Autodesk Fusion 360 part; units mm, degrees
sketch "Sketch1" plane through (0, 0, 0) normal (0, 0, 1) x (1, 0, 0)
  circle A0 centre (0, 0) radius 16.5
  circle A1 centre (0, 0) radius 15.5
  line L0 (-25, -5) -> (25, -5)
  line L1 (25, -5) -> (25, 5)
  line L2 (25, 5) -> (-25, 5)
  line L3 (-25, 5) -> (-25, -5)
  line L4 (-25, -5) -> (25, 5) construction
  line L5 (25, -5) -> (-25, 5) construction
  line L6 (-5, 25) -> (5, 25)
  line L7 (5, 25) -> (5, -25)
  line L8 (5, -25) -> (-5, -25)
  line L9 (-5, -25) -> (-5, 25)
  line L10 (-5, 25) -> (5, -25) construction
  line L11 (5, 25) -> (-5, -25) construction
  circle A2 centre (0, 4) radius 1
  circle A3 centre (0, -4) radius 1
  circle A4 centre (-3, 0) radius 1
  circle A5 centre (3, 0) radius 1
  dimension "d1" = 33
  dimension "d15" = 31
  dimension "d18" = 50
  dimension "d19" = 10
  dimension "d20" = 10
  dimension "d21" = 50
  dimension "d22" = 2
  dimension "d23" = 2
  dimension "d25" = 2
  dimension "d26" = 4
  dimension "d27" = 8
  dimension "d28" = 2
  dimension "d29" = 3
  dimension "d30" = 6
extrude "Extrude1" add sketch "Sketch1" along normal blind 37 contours A0 A1 L0 L2 | A0 A1 L2 L7 | A0 A1 L0 L7 | A0 A1 L7 L9 | A1 L2 L7 | A1 L0 L2 L7 | A0 A1 L7 L9 | A1 L0 L7 | A0 A1 L2 L9 | A1 L2 L7 L9 | A2 | A3 | L0 L2 L7 L9 | A0 A1 L0 L9 | A1 L0 L7 L9 | A0 A1 L0 L2 | A1 L2 L9 | A1 L0 L9 | A1 L0 L2 L9 | A4 | A5
sketch "Sketch2" plane through (0, 0, 0) normal (1, 0, 0) x (0, 0, -1)
  circle A0 centre (-39.9957, 0.4126) radius 20
  circle A1 centre (-39.9957, 0.4126) radius 17.5
  circle A2 centre (-39.9957, 0.4126) radius 16
  dimension "d4" = 40
  dimension "d7" = 35
  dimension "d10" = 32
extrude "Extrude2" add sketch "Sketch2" along normal blind 100 contours A0 | A1 | A2
extrude "Extrude3" add sketch "Sketch2" against normal blind 130 contours A1 | A2
extrude "Extrude4" cut sketch "Sketch2" along normal blind 140 and the other way blind 90 contours A2
extrude "Extrude5" cut sketch "Sketch1" along normal blind 40 contours A1 L2 L7 | A1 L0 L2 L7 | A1 L0 L7 | A1 L2 L7 L9 | A2 | A3 | L0 L2 L7 L9 | A1 L0 L7 L9 | A1 L2 L9 | A1 L0 L9 | A1 L0 L2 L9 | A4 | A5
extrude "Extrude6" add sketch "Sketch1" along normal blind 2 from surface at 3 contours A1 L0 L2 L7 | A1 L2 L7 L9 | L0 L2 L7 L9 | A1 L0 L7 L9 | A1 L0 L2 L9
For this review, take the finished solid that the model builds, in its own axes (mm). A direction names the side the tool comes from. Coordinates: 2 decimals unless noted, no trailing zeros. Order: outer loops, then holes, each group sorted by start corner. A loop starts at its lowest first (then second) coordinate and runs counter-clockwise, first axis right, second up. Notation, with made-up numbers: (-27.75, -34.75) - (-16.75, -34.75) arc R23 ccw to (-16.75, -0.75) - close; hole circle Ø1 at (-39.75, 12.5). An arc over 180 degrees is marked (long way). Answer as a JSON object with one key per item and string values. Group by question number.
1. We need section A-A on y = -11. State the section outline as (x, z) points, then the cut area to 3 significant figures.
2. For probe 1 along Y at (x, z) = (0, 3.5); probe 2 along X at (y, z) = (0, 9); probe 3 along Y at (x, z) = (-3, 4), list the stretches that pass through material, from the lowest coordinate up.
3. We need section C-C on x = 65.5. State the section outline as (y, z) points, then the cut area to 3 significant figures.
4. We need section D-D on y = 8. State the section outline as (x, z) points, then the cut area to 3 significant figures.
5. For faces 5 (the cylindrical face through (-12.16, -11.15, 13.56)), 6 (the cylindrical face through (49.3, -0.467, 59.976)), 7 (the cylindrical face through (-2.018, -15.368, 14.64)), list the 3-axis set-ups (+Z, -Z, +X, -X, +Y, -Y) from which the entire face can be reached by the end or side of a thin tool; tool diameter is ignored.
6. The part is to be moulded in two halves that separate along X. For faces 1 (the flat face through (100, 14, 49)), 2 (the flat face through (-15, -5, 0)), 3 (the flat face through (0, 0, 5)), 4 (the flat face through (0, 0, 3)), say which applies: pulls with the +X half, pulls with the -X half, needs draft (parallel to the pull), parting line crosses it, or undercut.
7. Clearance check with flat-ended pins moving along their axes: P1, Ø1, axis at x = -7.5, z = 4, coming from the -Y side; P2, Ø1, axis at x = 8.5, z = 3.5, coming from the -Y side; P3, Ø1, axis at y = -3.5, z = 14.5, coming from the +X side (3 decimals). State where each tip first meets the part, or that it passes through.
8. We need section B-B on z = 13. State the section outline as (x, y) points.
Final values:
{
 "1": {"outline": "(-130, 26.73) - (-12.3, 26.73) - (-12.3, 0) - (-10.92, 0) - (-10.92, 28.78) - (-90, 28.78) - (-90, 51.21) - (100, 51.21) - (100, 56.42) - (0, 56.42) - (0, 53.26) - (-130, 53.26) - close; (-5, 3) - (5, 3) - (5, 5) - (-5, 5) - close; (10.92, 0) - (12.3, 0) - (12.3, 23.57) - (100, 23.57) - (100, 28.78) - (10.92, 28.78) - close", "area": "2,480 mm²"},
 "2": {"probe 1": "-16.5 to -5, -3 to 3, 5 to 16.5", "probe 2": "-16.5 to -15.5, 15.5 to 16.5", "probe 3": "-16.22 to -1, 1 to 16.22"},
 "3": {"outline": "circle Ø40 at (0.41, 40); hole circle Ø32 at (0.41, 40)", "area": "452 mm²"},
 "4": {"outline": "(-130, 24.23) - (-14.43, 24.23) - (-14.43, 0) - (-13.28, 0) - (-13.28, 25.91) - (-90, 25.91) - (-90, 54.08) - (100, 54.08) - (100, 58.5) - (0, 58.5) - (0, 55.77) - (-130, 55.77) - close; (-5, 3) - (5, 3) - (5, 5) - (-5, 5) - close; (13.28, 0) - (14.43, 0) - (14.43, 21.49) - (100, 21.49) - (100, 25.91) - (13.28, 25.91) - close", "area": "2,440 mm²"},
 "5": {"face 5": "-Z", "face 6": "+X", "face 7": "none"},
 "6": {"face 1": "pulls with the +X half", "face 2": "needs draft", "face 3": "undercut", "face 4": "undercut"},
 "7": {"P1": "y = -14.94", "P2": "y = -14.43", "P3": "x = 16.225"},
 "8": {"outline": "circle Ø33 at (0, 0); hole circle Ø31 at (0, 0)"}
}
